Design review of the part built by this model. Coordinates are the model's own, in mm. A direction names the side the tool comes from. Coordinates: 2 decimals unless noted, no trailing zeros. Write each loop counter-clockwise with the first axis right and the second up, starting at its lowest first coordinate (ties: lowest second). Pieces come first, ordered by that corner, then holes.
Q1. Machinability: for faces 4 (the flat face through (-77.133, -121, 1)), 5 (the flat face through (-177, -121, 50.8)), 6 (the flat face through (104, -171.45, 2)), 7 (the flat face through (-177, -69.85, -1)), 8 (the flat face through (-1, -30, 177.8)), which of the approach directions +Z, -Z, +X, -X, +Y, -Y give a long, thin tool a straight path to every point of the face, cutting with its end or side? Answer none if there is none.
Q2. Insertion check: pin 1 (2.5 mm diameter, centred on x = -1, z = 183.5, fed in from +Y); pin 2 (10 mm diameter, centred on x = -111.5, z = 20, fed in from +Y); pin 3 (1.5 mm diameter, centred on y = -106.5, z = 129.5, fed in from +X) (3 decimals); pin 4 (9 mm diameter, centred on x = 26, z = -181, fed in from +Y). Each pin has a flat end and moves straight along its axis. Give the tip position at first contact, or say it passes through.
Q3. For probe 1 along Z at (x, y) = (23, 44); probe 2 along Y at (x, z) = (8, -101.6); probe 3 along X at (y, z) = (-101, -7) (3 decimals), list the stretches that pass through material, from the lowest coordinate up.
Q4. Mouldability with a two-part tool opening along X and no side actions: class faces 1 (the flat face through (-177, -121, -50.8)), 2 (the flat face through (53.975, -30, -2)), 3 (the flat face through (-76, -171.45, 2)) as pulls with the +X half, pulls with the -X half, needs draft (parallel to the pull), parting line crosses it, or undercut.
Q5. Take a section at B-B (y = 44.45). Give the boundary of the cut face in (x, z) (3 decimals), and give its area (3 significant figures).
Q6. Take a section at D-D (z = 162). Give the boundary of the cut face in (x, y) (3 decimals), and give its area (3 significant figures).
Q7. Take a section at C-C (z = -101.6). Give the boundary of the cut face in (x, y) (3 decimals), and give its area (3 significant figures).
Q8. Take a section at A-A (y = -76.5). Give the boundary of the cut face in (x, z) (3 decimals), and give its area (3 significant figures).
```python
from build123d import *

# Parameters (mm, degrees)
SKETCH1_W           = 355.6
SKETCH1_H           = 215.9
SKETCH1_R           = 38.1
BOSS_EXTRUDE1_DEPTH = 53.975
SKETCH4_W           = 107.95
SKETCH4_H           = 355.6
BOSS_EXTRUDE4_DEPTH = 63.5
SKETCH2_W           = 107.95
SKETCH2_H           = 355.6
BOSS_EXTRUDE5_DEPTH = 63.5
SKETCH3_W           = 101.6
SKETCH3_H           = 101.6
BOSS_EXTRUDE3_DEPTH = 101.6
SKETCH5_W           = 101.6
SKETCH5_H           = 101.6
BOSS_EXTRUDE6_DEPTH = 101.6


with BuildPart() as part:
    # Sketch1 → Boss-Extrude1 (new, symmetric)
    with BuildSketch(Plane(origin=(0, 0, 0), x_dir=(0, 0, -1), z_dir=(1, 0, 0))):
        Rectangle(SKETCH1_W, SKETCH1_H)
        with Locations((-101.6, 44.45)):
            Circle(SKETCH1_R, mode=Mode.SUBTRACT)
        with Locations((101.6, 44.45)):
            Circle(SKETCH1_R, mode=Mode.SUBTRACT)
    extrude(amount=BOSS_EXTRUDE1_DEPTH, both=True)

    # Sketch4 → Boss-Extrude4 (add)
    with BuildSketch(Plane.XZ.offset(107.95)):
        Rectangle(SKETCH4_W, SKETCH4_H)
    extrude(amount=BOSS_EXTRUDE4_DEPTH)

    # Sketch2 → Boss-Extrude5 (add)
    with BuildSketch(Plane.XZ.offset(171.45)):
        with BuildLine():
            Line((-53.975, -177.8), (-53.975, 177.8))
            ThreePointArc((-53.975, 177.8), (-185.812111083, 0), (-53.975, -177.8))
        make_face()
        Rectangle(SKETCH2_W, SKETCH2_H)
        with BuildLine():
            ThreePointArc((185.812111083, 0), (149.257075746, 110.672787824), (53.975, 177.8))
            Line((53.975, 177.8), (53.975, -177.8))
            ThreePointArc((53.975, -177.8), (149.257075746, -110.672787824), (185.812111083, 0))
        make_face()
        with BuildLine():
            ThreePointArc((-53.975, -177.8), (0, -185.812111083), (53.975, -177.8))
            Line((53.975, -177.8), (-53.975, -177.8))
        make_face()
        with BuildLine():
            Line((-53.975, 177.8), (53.975, 177.8))
            ThreePointArc((53.975, 177.8), (0, 185.812111083), (-53.975, 177.8))
        make_face()
    extrude(amount=BOSS_EXTRUDE5_DEPTH)

    # Sketch3 → Boss-Extrude3 (add)
    with BuildSketch(Plane(origin=(0, -171.45, 0), x_dir=(1, 0, 0), z_dir=(0, 1, 0))):
        with Locations((-127.933042902, 0)):
            Rectangle(SKETCH3_W, SKETCH3_H)
    extrude(amount=BOSS_EXTRUDE3_DEPTH)

    # Sketch5 → Boss-Extrude6 (add)
    with BuildSketch(Plane.ZY.offset(178.733042902)):
        with Locations((0, -120.65)):
            Rectangle(SKETCH5_W, SKETCH5_H)
    extrude(amount=BOSS_EXTRUDE6_DEPTH)


solid = part.part
```
Response:
1. face 4: +Z, -Z, +Y
1. face 5: +Z, -X, +Y
1. face 6: +Z, -Z, +X, +Y
1. face 7: +Z, -Z, -X, +Y
1. face 8: +Z, +X, -X, +Y
2. pin 1: stops at y = -171.45
2. pin 2: stops at y = -69.85
2. pin 3: stops at x = 53.975
2. pin 4: stops at y = 107.95
3. probe 1: z = -177.8 to -139.7, -63.5 to 63.5, 139.7 to 177.8
3. probe 2: y = -234.95 to 6.35, 82.55 to 107.95
3. probe 3: x = -280.333 to -77.133, -53.975 to 53.975
4. face 1: needs draft
4. face 2: pulls with the +X half
4. face 3: undercut
5. outline: (-53.975, -177.8) - (53.975, -177.8) - (53.975, -139.7) - (-53.975, -139.7) - close; (-53.975, -63.5) - (53.975, -63.5) - (53.975, 63.5) - (-53.975, 63.5) - close; (-53.975, 139.7) - (53.975, 139.7) - (53.975, 177.8) - (-53.975, 177.8) - close
5. area: 21,900 mm2
6. outline: (-91.006, -234.95) - (91.006, -234.95) - (91.006, -171.45) - (53.975, -171.45) - (53.975, 107.95) - (-53.975, 107.95) - (-53.975, -171.45) - (-91.006, -171.45) - close
6. area: 41,700 mm2
7. outline: (-155.575, -234.95) - (155.575, -234.95) - (155.575, -171.45) - (53.975, -171.45) - (53.975, 6.35) - (-53.975, 6.35) - (-53.975, -171.45) - (-155.575, -171.45) - close; (-53.975, 82.55) - (53.975, 82.55) - (53.975, 107.95) - (-53.975, 107.95) - close
7. area: 41,700 mm2
8. outline: (-280.333, -50.8) - (-77.133, -50.8) - (-77.133, 50.8) - (-280.333, 50.8) - close; (-53.975, -177.8) - (53.975, -177.8) - (53.975, 177.8) - (-53.975, 177.8) - close
8. area: 59,000 mm2
